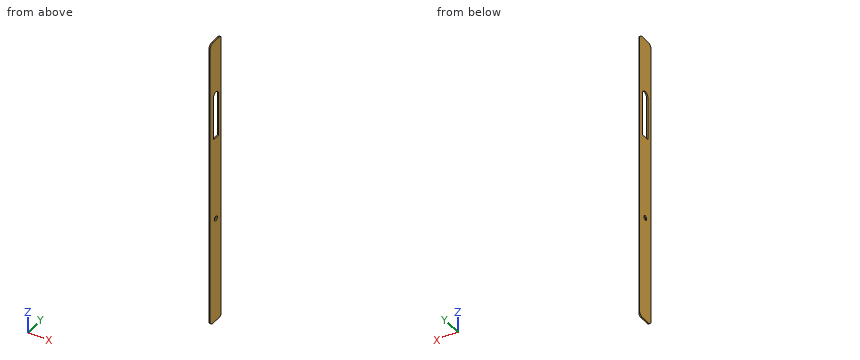
```python
from build123d import *

# Parameters (mm, degrees)
F0_W        = 8
F0_H        = 125
F1_DEPTH    = 0.5
F2_R        = 2
F3_R        = 1
F4_DEPTH    = 12.5
F5_T1_DEPTH = 125.3718610795


# Not quite as in the source:
# - a fillet or chamfer that OpenCascade refuses, or shapes differently, is made with other operations: its cross-section is extruded or revolved along the edge and cut away or added


with BuildPart() as f1:
    # F0 (on Right) → F1 (new body)
    with BuildSketch(Plane.YZ):
        with Locations((30.2877472714, 96.0264432559)):
            Rectangle(F0_W, F0_H)
    extrude(amount=F1_DEPTH)

    # F2
    f2_edges = [f1.edges().sort_by_distance(p)[0] for p in [
        (0.25, 26.287747, 158.526443),
        (0.25, 34.287747, 158.526443),
        (0.25, 34.287747, 33.526443),
        (0.25, 26.287747, 33.526443),
    ]]
    fillet(f2_edges, radius=F2_R)

    # F3 (on face) → F4 (cut, symmetric)
    with BuildSketch(Plane.YZ.offset(0.5)):
        with BuildLine():
            Line((28.4577472714, 133.5264432559), (28.4577472714, 115.0264432559))
            Line((28.4577472714, 115.0264432559), (32.1177472714, 115.0264432559))
            Line((32.1177472714, 115.0264432559), (32.1177472714, 133.5264432559))
            ThreePointArc((32.1177472714, 133.5264432559), (30.2877472714, 135.3564432559), (28.4577472714, 133.5264432559))
        make_face()
        with Locations((30.2877472714, 79.0264432559)):
            Circle(F3_R)
    extrude(amount=F4_DEPTH, both=True, mode=Mode.SUBTRACT)

    # F5: chamfer of 0.5 on 1 edges, made by hand

    # F5_s2 → F5_t1 (cut)
    with BuildSketch(Plane.XY.offset(33.3405127162)):
        Polygon((0.5, 33.7877472714), (0, 34.2877472714), (0.5, 34.2877472714), align=None)
    extrude(amount=F5_T1_DEPTH, mode=Mode.SUBTRACT)


solid = f1.part
```
Check sheet for the modelled part. Datum: model origin and axes. Units: mm. Give positions to 0.01 mm unless a question says otherwise; leave off trailing zeros. Order: outer loops, then holes, each group sorted by start corner. A loop starts at its lowest first (then second) coordinate and runs counter-clockwise, first axis right, second up. Notation, with made-up numbers: M -12.5,-22 L 4.5,-22 A6 cw 4.5,-17 Z; hole C -10,23 d8. An arc over 180 degrees is marked long. Answer in a Markdown table with one row per item.
1) Cross-section at B-B, the plane x = 0.4. Enter the section's corners in (y, z), plus the area to 3 significant figures.
Filled sheet:
| item | result |
|---|---|
| outline | M 26.29,35.53 A2 ccw 28.29,33.53 L 32.29,33.53 A2 ccw 33.89,34.33 L 33.89,157.73 A2 ccw 32.29,158.53 L 28.29,158.53 A2 ccw 26.29,156.53 Z; hole M 28.46,115.03 L 32.12,115.03 L 32.12,133.53 A1.83 ccw 28.46,133.53 Z; hole C 30.29,79.03 d2 |
| area | 871 mm2 |
2) Thickness scan on L1, parallel to Z at x = 0.05, y = 29.5; L2, parallel to Z at x = 0.3, y = 31; L3, parallel to Z at x = 0.35, y = 32.5. Record the ranges inside material, lowest first. Write a range as [from, to].
Filled sheet:
| item | result |
|---|---|
| L1 | z = [33.53, 78.41], [79.64, 115.03], [135.18, 158.53] |
| L2 | z = [33.53, 78.32], [79.73, 115.03], [135.21, 158.53] |
| L3 | z = [33.54, 158.52] |
3) Cross-section at C-C, the plane z = 68. Enter the section's corners in (x, y), plus the area to 4 significant figures.
Filled sheet:
| item | result |
|---|---|
| outline | M 0,26.29 L 0.5,26.29 L 0.5,33.79 L 0,34.29 Z |
| area | 3.875 mm2 |
4) Cross-section at A-A, the plane z = 123. Enter the section's corners in (x, y).
Filled sheet:
| item | result |
|---|---|
| outline | M 0,26.29 L 0.5,26.29 L 0.5,28.46 L 0,28.46 Z; M 0,32.12 L 0.5,32.12 L 0.5,33.79 L 0,34.29 Z |
